Geometry check sheet. Reference: the model listing, model coordinates, mm. A direction names the side the tool comes from. Coordinates: 2 decimals unless noted, no trailing zeros. Loops run counter-clockwise (first coordinate to the right, second up) from the corner with the lowest first, then second, coordinate; pieces in that order, holes last.
Autodesk Inventor part; units mm, degrees
ref_plane "YZ Plane" through (0, 0, 0) normal (1, 0, 0) x (0, 1, 0)
ref_plane "XZ Plane" through (0, 0, 0) normal (0, 1, 0) x (-1, 0, 0)
ref_plane "XY Plane" through (0, 0, 0) normal (0, 0, 1) x (1, 0, 0)
sketch "Sketch1" plane through (0, 0, 0) normal (0, 0, 1) x (1, 0, 0)
  line L0 (0, 0) -> (160, 0)
  line L1 (160, 0) -> (160, 160)
  line L2 (160, 160) -> (0, 160)
  line L3 (0, 160) -> (0, 0)
  dimension "d0" = 160
  dimension "d1" = 160
extrude "Extrusion1" add sketch "Sketch1" along normal blind 10
sketch "Sketch2" plane through (0, 0, 10) normal (0, 0, 1) x (1, 0, 0)
  line L0 (0, 0) -> (160, 0)
  line L1 (0, 0) -> (15, 0)
  line L2 (15, 0) -> (15, 15)
  line L3 (160, 160) -> (0, 160)
  line L4 (0, 160) -> (15, 160)
  line L5 (15, 160) -> (15, 145)
  line L6 (160, 0) -> (160, 160)
  line L7 (160, 160) -> (145, 160)
  line L8 (145, 160) -> (145, 143.5)
  line L9 (160, 0) -> (160, 15)
  line L10 (160, 15) -> (145, 15)
  circle A0 centre (15, 145) radius 7.5
  circle A1 centre (145, 143.5) radius 7.5
  circle A2 centre (145, 15) radius 7.5
  circle A3 centre (15, 15) radius 7.5
  dimension "d4" = 15
  dimension "d5" = 15
  dimension "d6" = 15
  dimension "d7" = 15
  dimension "d8" = 15
  dimension "d9" = 16.5
  dimension "d10" = 15
  dimension "d11" = 15
  dimension "d12" = 15
  dimension "d13" = 15
  dimension "d14" = 15
  dimension "d15" = 15
extrude "Extrusion2" cut sketch "Sketch2" against normal blind 10
sketch "Sketch3" plane through (0, 0, 10) normal (0, 0, 1) x (1, 0, 0)
  line L0 (0, 160) -> (0, 0)
  line L1 (0, 0) -> (80, 0)
  line L2 (0, 0) -> (160, 0)
  line L3 (80, 0) -> (0, 0)
  line L4 (0, 0) -> (80, 0)
  dimension "d18" = 80
  dimension "d19" = 80
  dimension "d20" = 80
sketch "Sketch4" plane through (0, 0, 10) normal (0, 0, 1) x (1, 0, 0)
  line L0 (0, 0) -> (160, 0)
  line L1 (0, 0) -> (0, 80)
  line L2 (0, 160) -> (0, 0)
  dimension "d21" = 80
sketch "Sketch5" plane through (0, 0, 10) normal (0, 0, 1) x (1, 0, 0)
  line L0 (0, 160) -> (0, 0)
  line L1 (0, 80) -> (80, 80)
  line L2 (84.0688, 89.1348) -> (89.9454, 81.0437)
  line L3 (89.9454, 81.0437) -> (85.8766, 71.9089)
  line L4 (85.8766, 71.9089) -> (75.9312, 70.8652)
  line L5 (75.9312, 70.8652) -> (70.0546, 78.9563)
  line L6 (70.0546, 78.9563) -> (74.1234, 88.0911)
  line L7 (74.1234, 88.0911) -> (84.0688, 89.1348)
  dimension "d22" = 80
  dimension "d23" = 10
extrude "Extrusion3" cut sketch "Sketch5" against normal blind 10
sketch "Sketch6" plane through (0, 0, 10) normal (0, 0, 1) x (1, 0, 0)
  line L0 (160, 0) -> (160, 160)
  line L1 (160, 0) -> (160, 80)
  point P0 (0, 0)
  dimension "d26" = 80
sketch "Sketch7" plane through (0, 0, 10) normal (0, 0, 1) x (1, 0, 0)
  line L0 (160, 0) -> (160, 160)
  line L1 (160, 80) -> (125, 80)
  circle A0 centre (125, 80) radius 7.5
  point P0 (0, 0)
  dimension "d27" = 35
  dimension "d28" = 15
extrude "Extrusion4" cut sketch "Sketch7" against normal blind 10
properties part number "101"
1) Section check A-A on y = 15. Record the cut outline in (x, z).
Data:
outline: (0, 0) - (7.5, 0) - (7.5, 10) - (0, 10) - close; (22.5, 0) - (137.5, 0) - (137.5, 10) - (22.5, 10) - close; (152.5, 0) - (160, 0) - (160, 10) - (152.5, 10) - close
2) Section check C-C on z = 7.5. Record the cut outline in (x, y).
Data:
outline: (0, 0) - (160, 0) - (160, 160) - (0, 160) - close; hole circle Ø15 at (15, 15); hole circle Ø15 at (15, 145); hole (70.05, 78.96) - (75.93, 70.87) - (85.88, 71.91) - (89.95, 81.04) - (84.07, 89.13) - (74.12, 88.09) - close; hole circle Ø15 at (125, 80); hole circle Ø15 at (145, 15); hole circle Ø15 at (145, 143.5)
3) Depth check by flat-ended pin: pin 1 (13.5 mm diameter, centred on x = 15, y = 145, fed in from +Z). Enter the tip coordinate at first touch or a pass-through.
Data:
pin 1: passes through
4) Mould release check, pull along X, two halves, no side actions. Record for faces 1 (the flat face through (81, 160, 5)), 2 (the cylindrical face through (152.154, 17.253, 5.07)), 3 (the flat face through (160, 79, 5)): +X half, -X half, draft (parallel to the pull), parting line (faces both ways), or undercut.
Data:
face 1: draft
face 2: undercut
face 3: +X half
5) Access from +Z, -Z, +X, -X, +Y, -Y to the whole of each face (thin tool, end or side, straight path). Record for faces 4 (the flat face through (61, 81, 0)), 5 (the flat face through (87.94, 76.54, 5.07)).
Data:
face 4: -Z, +X, -X, +Y, -Y
face 5: +Z, -Z
6) Material ranges on probe 1 along Y at (x, z) = (15, 2.5); probe 2 along Y at (x, z) = (145, 7.25); probe 3 along X at (y, z) = (145, 7.5), recorded low to high.
Data:
probe 1: y = 0 to 7.5, 22.5 to 137.5, 152.5 to 160
probe 2: y = 0 to 7.5, 22.5 to 136, 151 to 160
probe 3: x = 0 to 7.5, 22.5 to 137.65, 152.35 to 160
